Can you work these out from the model? Positions are in its coordinate system, mm. A direction names the side the tool comes from. Give positions to 0.01 mm unless a question says otherwise; leave off trailing zeros. Order: outer loops, then holes, each group sorted by start corner. A loop starts at its lowest first (then second) coordinate and runs counter-clockwise, first axis right, second up. Notation, with made-up numbers: (49.25, 43.5) - (105.25, 43.5) arc R13 ccw to (105.25, 48.5) - close; hole circle Ø10 at (87.5, 85). An arc over 180 degrees is marked (long way). Write each question's results on one line, items separated by ' | '. Start each with the question number.
from build123d import *

# Parameters (mm, degrees)
SKETCH1_W           = 150
SKETCH1_H           = 150
BOSS_EXTRUDE1_DEPTH = 10
SKETCH2_R           = 50
BOSS_EXTRUDE2_DEPTH = 60
SKETCH3_R           = 60
BOSS_EXTRUDE3_DEPTH = 10
SKETCH7_W           = 150
SKETCH7_H           = 60
BOSS_EXTRUDE6_DEPTH = 30
SKETCH8_R           = 10
CUT_EXTRUDE2_DEPTH  = 20
FILLET3_R           = 10
FILLET4_R           = 3
CHAMFER1_SIZE       = 10
BOSS_EXTRUDE7_DEPTH = 3
CIRPATTERN1_COUNT   = 4


with BuildPart() as part:
    # Sketch1 → Boss-Extrude1 (new body)
    with BuildSketch(Plane(origin=(0, 0, 0), x_dir=(1, 0, 0), z_dir=(0, 1, 0))):
        Rectangle(SKETCH1_W, SKETCH1_H)
    extrude(amount=BOSS_EXTRUDE1_DEPTH)

    # Sketch2 → Boss-Extrude2 (add)
    with BuildSketch(Plane(origin=(0, 10, 0), x_dir=(1, 0, 0), z_dir=(0, 1, 0))):
        with Locations(Location((0, 0, 0), (0, 0, 270))):
            Circle(SKETCH2_R)
    extrude(amount=BOSS_EXTRUDE2_DEPTH)

    # Sketch3 → Boss-Extrude3 (add)
    with BuildSketch(Plane(origin=(0, 70, 0), x_dir=(1, 0, 0), z_dir=(0, 1, 0))):
        with Locations(Location((0, 0, 0), (0, 0, 270))):
            Circle(SKETCH3_R)
    extrude(amount=BOSS_EXTRUDE3_DEPTH)

    # Sketch7 → Boss-Extrude6 (add)
    with BuildSketch(Plane(origin=(0, 0, 0), x_dir=(-1, 0, 0), z_dir=(0, -1, 0))):
        Rectangle(SKETCH7_W, SKETCH7_H)
    extrude(amount=-BOSS_EXTRUDE6_DEPTH)

    # Sketch8 → Cut-Extrude2 (cut)
    with BuildSketch(Plane(origin=(0, 80, 0), x_dir=(1, 0, 0), z_dir=(0, 1, 0))):
        with Locations(Location((0, 0, 0), (0, 0, 270))):
            Circle(SKETCH8_R)
    extrude(amount=-CUT_EXTRUDE2_DEPTH, mode=Mode.SUBTRACT)

    # Fillet3
    fillet3_edges = [part.edges().sort_by_distance(p)[0] for p in [
        (0, 70, -60),
    ]]
    fillet(fillet3_edges, radius=FILLET3_R - 0.0001)  # a hair under: the kernel refuses the full size

    # Fillet4
    fillet4_edges = [part.edges().sort_by_distance(p)[0] for p in [
        (75, 5, 75),
        (-75, 5, 75),
        (-75, 5, -75),
        (75, 5, -75),
    ]]
    fillet(fillet4_edges, radius=FILLET4_R)

    # Chamfer1
    chamfer1_edges = [part.edges().sort_by_distance(p)[0] for p in [
        (75, 30, 0),
        (-75, 30, 0),
    ]]
    chamfer(chamfer1_edges, length=CHAMFER1_SIZE)

    # Sketch9 → Boss-Extrude7 (add)
    with BuildSketch(Plane(origin=(0, 10, 0), x_dir=(1, 0, 0), z_dir=(0, 1, 0))):
        Polygon((-57.993107668, -63.993107668), (-60.993107668, -58.796955246), (-66.993107668, -58.796955246), (-69.993107668, -63.993107668), (-66.993107668, -69.189260091), (-60.993107668, -69.189260091), align=None)
    boss_extrude7 = extrude(amount=BOSS_EXTRUDE7_DEPTH)

    # CirPattern1: Boss-Extrude7 ×4 about axis
    cirpattern1_axis = Axis((0, 0, 0), (0, 1, 0))
    for i in range(1, CIRPATTERN1_COUNT):
        add(boss_extrude7.rotate(cirpattern1_axis, i * 360 / CIRPATTERN1_COUNT))


solid = part.part
Q1. Will these pins go through, and if not, where does the flat tip stop? P1, Ø2.5, axis at y = 12, z = -63, coming from the -X side; P2, Ø8.5, axis at x = -64, z = -64.5, coming from the +Y side; P3, Ø4, axis at x = 43, y = 38, coming from the -Z side.
Q2. If I drill on probe 1 along Z at (x, y) = (-64, 29); probe 2 along Y at (x, z) = (-62, 0.5); probe 3 along X at (y, z) = (68, 0), over which ranges is the centre line in solid material (lowest first)? Write a range as from..to.
Q3. If we section it at C-C (y = 47.5): Please give me the cut outline in (x, z).
Q4. Which directions (+Z, -Z, +X, -X, +Y, -Y) give clear straight access to the entire face, cutting with the end or side of a thin tool? Please do faces 1 (the flat face through (-1, 10, 52)), 2 (the flat face through (-64, 13, -64)), 3 (the flat face through (64, 13, 64)), 4 (the flat face through (-75, 8, 1)), 5 (the flat face through (-1, 5, -75)).
Q5. Thinking about a two-plate mould opening in X: for faces 6 (the cylindrical face through (-9.76, 70.14, -2.17)), 7 (the flat face through (-70, 25, 0)), 8 (the flat face through (1, 80, 12)), 9 (the flat face through (75, 8, 1)), which applies, released by +X, released by -X, zero draft, split by the parting line, or undercut?
Findings below:
1) P1: stops at x = -69.19 | P2: stops at y = 13 | P3: stops at z = -28.62
2) probe 1: z = -30..30 | probe 2: y = 0..30 | probe 3: x = -50..-10, 10..50
3) outline: circle Ø100 at (0, 0)
4) face 1: none | face 2: -Z, +X, -X, +Y | face 3: +Z, +X, -X, +Y | face 4: +Z, -Z, -X, +Y, -Y | face 5: -Z, +X, -X, +Y, -Y
5) face 6: undercut | face 7: released by -X | face 8: zero draft | face 9: released by +X
